from build123d import *

# Parameters (mm, degrees)
SKETCH2_R           = 12.7
BOSS_EXTRUDE1_DEPTH = 127


with BuildPart() as part:
    # Sketch2 → Boss-Extrude1 (new body)
    with BuildSketch(Plane(origin=(0, 0, 0), x_dir=(1, 0, 0), z_dir=(0, 1, 0))):
        Circle(SKETCH2_R)
    extrude(amount=BOSS_EXTRUDE1_DEPTH)

    # Sketch4 → 1/4-20 Tapped Hole1 (revolve, cut)
    with BuildSketch(Plane(origin=(0.473892963, 127, 0.332854466), x_dir=(0, 0, 1), z_dir=(1, 0, 0))):
        Polygon((0, 0), (0, 33.283816902), (2.5527, 31.75), (2.5527, 0), align=None)
    f_1_4_20_tapped_hole1 = revolve(axis=Axis((0.473892963, 133.35, 0.332854466), (0, -1, 0)), mode=Mode.SUBTRACT)

    # Mirror1: 1/4-20 Tapped Hole1 across plane
    add(f_1_4_20_tapped_hole1.mirror(Plane.ZX.offset(63.5)), mode=Mode.SUBTRACT)


solid = part.part
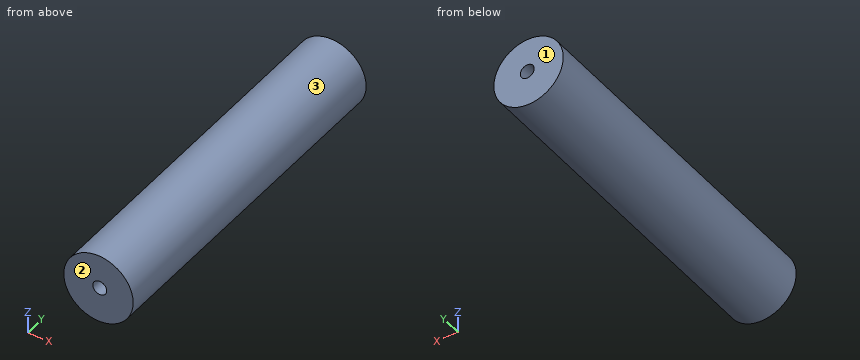
Work out the finished part from the listing and answer in its coordinate system (mm). Face numbers are marked on the shaded views. Coordinates: 2 decimals unless noted, no trailing zeros. Write each loop counter-clockwise with the first axis right and the second up, starting at its lowest first coordinate (ties: lowest second). Pieces come first, ordered by that corner, then holes. Notation, with made-up numbers: M 76.25,59.25 L 101.25,59.25 A18 ccw 101.25,77.25 Z; hole C 9.5,-34.75 d10. An arc over 180 degrees is marked long. Answer as CSV lines item,"result". Start each with the question number.
Item 1: Determine the mould class of the marked faces 1, 2 and 3 for opening direction Y: released by +Y, released by -Y, zero draft, split by the parting line, or undercut.
Item 2: Section C-C on x = -6 is taken. Write down the section's boundary in (y, z).
Item 3: Section D-D on y = 112 is taken. Write down the section's boundary in (x, z), and give its area (3 significant figures).
Item 4: Consider L1, parallel to X at y = 26, z = -2; L2, parallel to X at y = 109, z = -2.5; L3, parallel to X at y = 74.5, z = 4.5. Determine where each line is inside the solid, lowest interval first.
Item 5: Flat-ended cylindrical pins translate along their axes: P1, Ø12, axis at x = 0.5, y = 66, coming from the +Z side; P2, Ø3, axis at x = 6.5, y = 23, coming from the +Z side; P3, Ø1, axis at x = 3, y = 97.5, coming from the -Z side; P4, Ø10, axis at y = 54, z = -7, coming from the -X side. Find the tip coordinate at first contact, or state that the pin passes through.
Item 6: Section A-A on y = 70.5 is taken. Write down the section's boundary in (x, z), and give its area (3 significant figures).
Item 7: Section B-B on z = -4 is taken. Write down the section's boundary in (x, y).
Checks:
1,face 1,"released by +Y"
1,face 2,"released by -Y"
1,face 3,"zero draft"
2,outline,"M 0,-11.19 L 127,-11.19 L 127,11.19 L 0,11.19 Z"
3,outline,"C 0,0 d25.4; hole C 0.47,0.33 d5.11"
3,area,"486 mm²"
4,L1,"x = -12.54 to -0.56, 1.51 to 12.54"
4,L2,"x = -12.45 to 12.45"
4,L3,"x = -11.88 to 11.88"
5,P1,"stops at z = 12.7"
5,P2,"stops at z = 11.67"
5,P3,"stops at z = -12.45"
5,P4,"stops at x = -12.54"
6,outline,"C 0,0 d25.4"
6,area,"507 mm²"
7,outline,"M -12.05,0 L 12.05,0 L 12.05,127 L -12.05,127 Z"
